from build123d import *

# Parameters (mm, degrees)
SKETCH_1_W          = 30
SKETCH_1_H          = 60
SKETCH_1_R          = 3.25
EXTRUDE_1_DEPTH     = 6
SKETCH_2_W          = 2
SKETCH_2_H          = 20
CUT_EXTRUDE_1_DEPTH = 31
CHAMFER_2_SIZE      = 5
CHAMFER_2_SIZE2     = 2.886751346
CHAMFER_3_SIZE      = 5
CHAMFER_3_SIZE2     = 2.886751346
CHAMFER_4_SIZE      = 0.5


with BuildPart() as part:
    # Эскиз1 → Бобышка-Вытянуть1 (new body)
    with BuildSketch(Plane.XY):
        Rectangle(SKETCH_1_W, SKETCH_1_H)
        with Locations((0, -20)):
            Circle(SKETCH_1_R, mode=Mode.SUBTRACT)
        Circle(SKETCH_1_R, mode=Mode.SUBTRACT)
    extrude(amount=EXTRUDE_1_DEPTH)

    # Эскиз2 → Вырез-Вытянуть1 (cut, through all)
    with BuildSketch(Plane.ZY.offset(-15)):
        with Locations((5, 20)):
            Rectangle(SKETCH_2_W, SKETCH_2_H)
    extrude(amount=CUT_EXTRUDE_1_DEPTH, mode=Mode.SUBTRACT)

    # Фаска2
    chamfer_2_edges = [part.edges().sort_by_distance(p)[0] for p in [
        (-15, 30, 2),
    ]]
    chamfer_2_side = [part.faces().sort_by_distance(p)[0] for p in [
        (-15, -2.5, 2.75),
    ]]
    chamfer(chamfer_2_edges, length=CHAMFER_2_SIZE, length2=CHAMFER_2_SIZE2, reference=chamfer_2_side[0])

    # Фаска3
    chamfer_3_edges = [part.edges().sort_by_distance(p)[0] for p in [
        (15, 30, 2),
    ]]
    chamfer_3_side = [part.faces().sort_by_distance(p)[0] for p in [
        (15, -2.5, 2.75),
    ]]
    chamfer(chamfer_3_edges, length=CHAMFER_3_SIZE, length2=CHAMFER_3_SIZE2, reference=chamfer_3_side[0])

    # Фаска4
    chamfer_4_edges = [part.edges().sort_by_distance(p)[0] for p in [
        (-3.25, -20, 0),
        (-3.25, -20, 6),
        (-3.25, 0, 0),
        (-3.25, 0, 6),
    ]]
    chamfer(chamfer_4_edges, length=CHAMFER_4_SIZE)


solid = part.part
Verification items for the finished model (mm, model axes). A direction names the side the tool comes from. Coordinates: 2 decimals unless noted, no trailing zeros. Order: outer loops, then holes, each group sorted by start corner. A loop starts at its lowest first (then second) coordinate and runs counter-clockwise, first axis right, second up. Notation, with made-up numbers: M 39,38.25 L 56,38.25 A8 cw 56,48.25 Z; hole C 18.25,-30.75 d8. An arc over 180 degrees is marked long. One line per item, written item: value. Start each with the question number.
Item 1: Thickness scan on probe 1 along Y at (x, z) = (0, 1.65); probe 2 along Y at (x, z) = (-2.5, 2.9); probe 3 along Z at (x, y) = (-5.75, 14). Record the ranges inside material, lowest first.
Item 2: Sectioned sample at A-A on y = -20. Record the cut outline in (x, z), then the cut area to 4 significant figures.
Item 3: Sectioned sample at C-C on z = 1.2. Record the cut outline in (x, y).
Item 4: Mould release check, pull along Y, two halves, no side actions. Record for faces 3 (the flat face through (13.536, 27.535, 1.972)), 4 (the cylindrical face through (-0.423, -16.778, 2.965)), 5 (the flat face through (0, -30, 3)), 6 (the flat face through (0, -10, 6)): pulls with the +Y half, pulls with the -Y half, needs draft (parallel to the pull), parting line crosses it, or undercut.
Item 5: Sectioned sample at B-B on x = 0. Record the cut outline in (y, z).
Item 6: Depth check by flat-ended pin: P1, Ø0.6, axis at x = 0, z = 5, coming from the +Y side; P2, Ø8, axis at x = -2.5, y = -20.5, coming from the +Z side. Enter the tip coordinate at first touch or a pass-through.
Item 7: Access from +Z, -Z, +X, -X, +Y, -Y to the whole of each face (thin tool, end or side, straight path). Record for faces 1 (the flat face through (0, 20, 4)), 2 (the flat face through (0, 30, 2)).
Item 8: Sectioned sample at D-D on y = 12. Record the cut outline in (x, z), then the cut area to 3 significant figures.
Calculated:
1. probe 1: -30 to -23.25, -16.75 to -3.25, 3.25 to 30
1. probe 2: -30 to -22.08, -17.92 to -2.08, 2.08 to 30
1. probe 3: 0 to 4
2. outline: M -15,0 L -3.75,0 L -3.25,0.5 L -3.25,5.5 L -3.75,6 L -15,6 Z; M 3.25,0.5 L 3.75,0 L 15,0 L 15,6 L 3.75,6 L 3.25,5.5 Z
2. area: 140.5 mm^2
3. outline: M -15,-30 L 15,-30 L 15,25 L 12.11,30 L -12.11,30 L -15,25 Z; hole C 0,-20 d6.5; hole C 0,0 d6.5
4. face 3: pulls with the +Y half
4. face 4: undercut
4. face 5: pulls with the -Y half
4. face 6: needs draft
5. outline: M -30,0 L -23.75,0 L -23.25,0.5 L -23.25,5.5 L -23.75,6 L -30,6 Z; M -16.75,0.5 L -16.25,0 L -3.75,0 L -3.25,0.5 L -3.25,5.5 L -3.75,6 L -16.25,6 L -16.75,5.5 Z; M 3.25,0.5 L 3.75,0 L 30,0 L 30,4 L 10,4 L 10,6 L 3.75,6 L 3.25,5.5 Z
6. P1: y = 10
6. P2: z = 6
7. face 1: +Z, +X, -X, +Y
7. face 2: +Z, -Z, +X, -X, +Y
8. outline: M -15,0 L 15,0 L 15,4 L -15,4 Z
8. area: 120 mm^2
